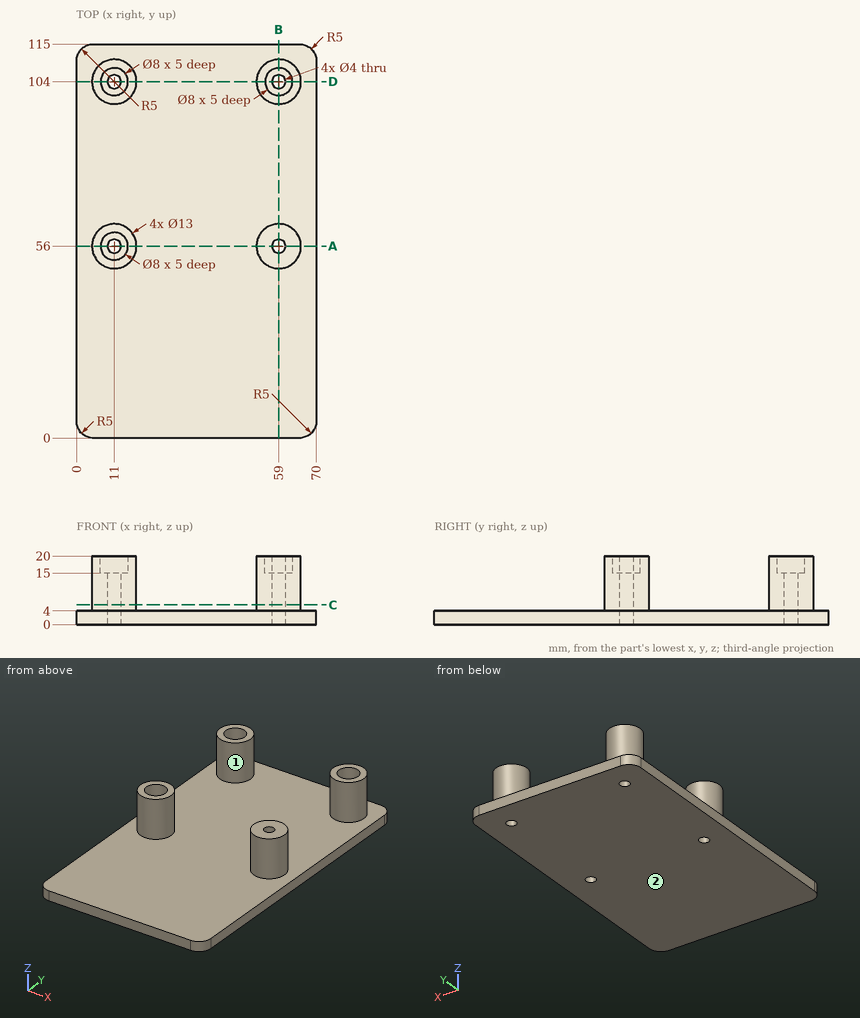
Study the drawing (mm; zero at the part's minimum x, y, z) and answer. Round coordinates to 2 decimals unless told otherwise and drop trailing zeros. Write each loop counter-clockwise with the first axis right and the second up, starting at its lowest first coordinate (ties: lowest second). Pieces come first, ordered by that corner, then holes.
Q1. Find section C-C on z = 5.75. Determine the outline of the cut face in (x, y).
Values:
outline: circle Ø13 at (11, 56); circle Ø13 at (11, 104); circle Ø13 at (59, 56); circle Ø13 at (59, 104); hole circle Ø4 at (11, 56); hole circle Ø4 at (11, 104); hole circle Ø4 at (59, 56); hole circle Ø4 at (59, 104)
Q2. Straight lines are drawn through the part: line 1 (Y direction, x = 11, z = 5.5); line 2 (Y direction, x = 11, z = 18.3); line 3 (Z direction, x = 27.5, y = 64). For each, find the intervals that lie inside material, in ascending order.
Values:
line 1: y = 49.5 to 54, 58 to 62.5, 97.5 to 102, 106 to 110.5
line 2: y = 49.5 to 52, 60 to 62.5, 97.5 to 100, 108 to 110.5
line 3: z = 0 to 4
Q3. The mould has two halves that part along X. Classify the marked faces 1 and 2: released by +X, released by -X, zero draft, split by the parting line, or undercut.
Values:
face 1: undercut
face 2: zero draft
Q4. Find section B-B on x = 59. Determine the outline of the cut face in (y, z).
Values:
outline: (0, 0) - (54, 0) - (54, 20) - (49.5, 20) - (49.5, 4) - (0, 4) - close; (58, 0) - (102, 0) - (102, 15) - (100, 15) - (100, 20) - (97.5, 20) - (97.5, 4) - (62.5, 4) - (62.5, 20) - (58, 20) - close; (106, 0) - (115, 0) - (115, 4) - (110.5, 4) - (110.5, 20) - (108, 20) - (108, 15) - (106, 15) - close
Q5. Flat-ended cylindrical pins translate along their axes: P1, Ø4, axis at x = 12, y = 54.5, coming from the +Z side; P2, Ø8, axis at x = 11.5, z = 16, coming from the -Y side; P3, Ø5, axis at y = 63, z = 11, coming from the -X side; P4, Ø2.5, axis at x = 59, y = 56, coming from the +Z side. Find the tip coordinate at first contact, or state that the pin passes through.
Values:
P1: stops at z = 15
P2: stops at y = 49.5
P3: stops at x = 6.31
P4: passes through
Q6. Find section D-D on y = 104. Determine the outline of the cut face in (x, z).
Values:
outline: (0, 0) - (9, 0) - (9, 15) - (7, 15) - (7, 20) - (4.5, 20) - (4.5, 4) - (0, 4) - close; (13, 0) - (57, 0) - (57, 15) - (55, 15) - (55, 20) - (52.5, 20) - (52.5, 4) - (17.5, 4) - (17.5, 20) - (15, 20) - (15, 15) - (13, 15) - close; (61, 0) - (70, 0) - (70, 4) - (65.5, 4) - (65.5, 20) - (63, 20) - (63, 15) - (61, 15) - close
Q7. Find section A-A on y = 56. Determine the outline of the cut face in (x, z), and give its area (3 significant figures).
Values:
outline: (0, 0) - (9, 0) - (9, 15) - (7, 15) - (7, 20) - (4.5, 20) - (4.5, 4) - (0, 4) - close; (13, 0) - (57, 0) - (57, 20) - (52.5, 20) - (52.5, 4) - (17.5, 4) - (17.5, 20) - (15, 20) - (15, 15) - (13, 15) - close; (61, 0) - (70, 0) - (70, 4) - (65.5, 4) - (65.5, 20) - (61, 20) - close
area: 516 mm2
